```python
from build123d import *

# Parameters (mm, degrees)
SKETCH_1_R          = 100
EXTRUDE_1_DEPTH     = 10
SKETCH_2_W          = 140
SKETCH_2_H          = 100
EXTRUDE_2_DEPTH     = 160.00000000000009
FILLET_1_R          = 70
FILLET_2_R          = 70
SKETCH_3_R          = 50
CUT_EXTRUDE_1_DEPTH = 160.00000000000009
CUT_EXTRUDE_START   = -1
SKETCH_13_R         = 9.999999999999998
CUT_EXTRUDE_5_DEPTH = 25
SKETCH_9_W          = 53.30531277978001
SKETCH_9_H          = 9.28529014360771
EXTRUDE_3_DEPTH     = 100
SKETCH_14_R         = 50
CUT_EXTRUDE_6_DEPTH = 7.7
SKETCH_15_W         = 17.036633895131082
SKETCH_15_H         = 20
CUT_EXTRUDE_7_DEPTH = 110.00000000000001
SKETCH_16_R         = 2.0000000000000036
SKETCH_16_R_2       = 2.000000000000005
SKETCH_16_R_3       = 2.0000000000000013
SKETCH_16_R_4       = 2.0000000000000027
SKETCH_16_R_5       = 2.0000000000000044
CUT_EXTRUDE_8_DEPTH = 10


with BuildPart() as part:
    # 草图1 → 凸台-拉伸1 (new body)
    with BuildSketch(Plane(origin=(0, 0, 0), x_dir=(1, 0, 0), z_dir=(0, 1, 0))):
        with Locations(Location((0, 0, 0), (0, 0, 270))):
            Circle(SKETCH_1_R)
    extrude(amount=EXTRUDE_1_DEPTH)

    # 草图2 → 凸台-拉伸2 (add)
    with BuildSketch(Plane(origin=(0, 0, 0), x_dir=(1, 0, 0), z_dir=(0, 1, 0))):
        Rectangle(SKETCH_2_W, SKETCH_2_H)
    extrude(amount=-EXTRUDE_2_DEPTH)

    # 圆角1
    fillet_1_edges = [part.edges().sort_by_distance(p)[0] for p in [
        (-70.00000000000001, -160.00000000000009, 7.11e-15),
    ]]
    fillet(fillet_1_edges, radius=FILLET_1_R)

    # 圆角2
    fillet_2_edges = [part.edges().sort_by_distance(p)[0] for p in [
        (69.99999999999999, -160.00000000000009, 7.11e-15),
    ]]
    fillet(fillet_2_edges, radius=FILLET_2_R - 0.0001)  # a hair under: the kernel refuses the full size

    # 草图3 → 切除-拉伸1 (cut)
    with BuildSketch(Plane(origin=(0, 0, -49.99999999999999), x_dir=(-1, 0, 0), z_dir=(0, 0, -1))):
        with Locations((0, -90)):
            Circle(SKETCH_3_R)
    extrude(amount=-CUT_EXTRUDE_1_DEPTH, mode=Mode.SUBTRACT)

    # 草图13 → 切除-拉伸5 (cut)
    with BuildSketch(Plane.ZY.offset(70.00000000000001).offset(CUT_EXTRUDE_START)):
        with Locations((6.94e-15, -90.00000000000009)):
            Circle(SKETCH_13_R)
    extrude(amount=-CUT_EXTRUDE_5_DEPTH, mode=Mode.SUBTRACT)

    # 草图9 → 凸台-拉伸3 (add)
    with BuildSketch(Plane(origin=(0, 0, -49.99999999999999), x_dir=(-1, 0, 0), z_dir=(0, 0, -1))):
        with Locations((0.3436291461197136, -140.89264507180383)):
            Rectangle(SKETCH_9_W, SKETCH_9_H)
        Polygon((-23.87404930056264, -43.75), (22.298543315194763, -43.75), (22.298543315194763, -37.81707315136096), (-23.87404930056264, -37.817073151360965), align=None)
    extrude(amount=-EXTRUDE_3_DEPTH)

    # 草图14 → 切除-拉伸6 (cut)
    with BuildSketch(Plane(origin=(0, 0, -49.99999999999999), x_dir=(-1, 0, 0), z_dir=(0, 0, -1))):
        with Locations((0, -90)):
            Circle(SKETCH_14_R)
    extrude(amount=-CUT_EXTRUDE_6_DEPTH, mode=Mode.SUBTRACT)

    # 草图15 → 切除-拉伸7 (cut)
    with BuildSketch(Plane(origin=(0, 10, 0), x_dir=(1, 0, 0), z_dir=(0, 1, 0))):
        with Locations((-60.48168305243448, -7.11e-15)):
            Rectangle(SKETCH_15_W, SKETCH_15_H)
    extrude(amount=-CUT_EXTRUDE_7_DEPTH, mode=Mode.SUBTRACT)

    # 草图16 → 切除-拉伸8 (cut)
    with BuildSketch(Plane(origin=(0, 10, 0), x_dir=(1, 0, 0), z_dir=(0, 1, 0))):
        with Locations(Location((10.537986720028217, 13.656988536588477, 0), (0, 0, 270))):
            Circle(SKETCH_16_R)
        with Locations(Location((17.09629237189259, -2.2976699359932877, 0), (0, 0, 270))):
            Circle(SKETCH_16_R_2)
        with Locations(Location((6.558305651864305, -15.954658472581762, 0), (0, 0, 270))):
            Circle(SKETCH_16_R_3)
        with Locations(Location((-10.537986720028309, -13.656988536588404, 0), (0, 0, 270))):
            Circle(SKETCH_16_R_4)
        with Locations(Location((-17.09629237189257, 2.2976699359934125, 0), (0, 0, 270))):
            Circle(SKETCH_16_R_4)
        with Locations(Location((-6.558305651864193, 15.954658472581803, 0), (0, 0, 270))):
            Circle(SKETCH_16_R_5)
    extrude(amount=-CUT_EXTRUDE_8_DEPTH, mode=Mode.SUBTRACT)


solid = part.part
```
Source: CAD feature listing. Evaluate the final solid. Frame: model axes, mm. A direction names the side the tool comes from. Give positions to 0.01 mm unless a question says otherwise; leave off trailing zeros. Loops run counter-clockwise (first coordinate to the right, second up) from the corner with the lowest first, then second, coordinate; pieces in that order, holes last. Notation, with made-up numbers: (39.5, -8) -> (88.5, -8) arc R31 cw to (88.5, 24) -> close; hole circle Ø5 at (76, 88). An arc over 180 degrees is marked (long way). Use a Markdown table: item, result. Add a question column.
(1) Ray query, line 1 (Z direction, x = -50.7, y = -90); line 2 (Y direction, x = 17, z = 68); line 3 (Y direction, x = -49.7, z = 0). Return the intervals inside material, ascending.
(2) Pull-direction query (Y, two-part tool) for faces 1 (the face through (32, -43, -50)), 2 (the face through (-51, -90, -10)), 3 (the face through (0, -43.75, 3)), 4 (the face through (1, 10, -1)); classes: +Y half, -Y half, draft (parallel to the pull), parting line (faces both ways), or undercut.
(3) Section query B-B (x = 39). Output: boundary loops of the cut face in (y, z), then the cut area to 3 significant figures.
(4) First-contact query: pin 1 Ø2.5 at (x, z) = (-17.1, -2.3) entering from +Y; pin 2 Ø10 at (y, z) = (-118, -33.5) entering from +X; pin 3 Ø3 at (x, y) = (27.5, -130) entering from -Z. Flat tips, straight axial feed; report the tip coordinate or a pass-through.
(5) Access query for faces 5 (the face through (70, -44, 1)), 6 (the face through (-1, -43, 50)), 7 (the face through (0, -136.25, 3)), 8 (the face through (-61, -100, 0)). Directions: +Z, -Z, +X, -X, +Y, -Y. A direction counts if a zero-diameter tool reaches every point of the face in a straight line with its end or side. Return the directions, or none.
(6) Section query A-A (y = -36). Output: boundary loops of the cut face in (x, z), then the cut area to 3 significant figures.
(7) Section query D-D (y = -106.5). Output: boundary loops of the cut face in (x, z).
Checked values:
| question | item | result |
|---|---|---|
| 1 | line 1 | -50 to -10, 10 to 50 |
| 1 | line 2 | 0 to 10 |
| 1 | line 3 | -139.29 to -100, -80 to 10 |
| 2 | face 1 | draft |
| 2 | face 2 | undercut |
| 2 | face 3 | undercut |
| 2 | face 4 | +Y half |
| 3 | outline | (-148.13, -50) -> (-121.29, -50) -> (-121.29, 50) -> (-148.13, 50) -> close; (-58.71, -50) -> (0, -50) -> (0, -92.08) -> (10, -92.08) -> (10, 92.08) -> (0, 92.08) -> (0, 50) -> (-58.71, 50) -> close |
| 3 | area | 10,400 mm^2 |
| 4 | pin 1 | y = 0 |
| 4 | pin 2 | x = 66.11 |
| 4 | pin 3 | z = -50 |
| 5 | face 5 | +Z, -Z, +X, -Y |
| 5 | face 6 | +Z, +X, -X, -Y |
| 5 | face 7 | +Z, -Z |
| 5 | face 8 | +Y |
| 6 | outline | (-70, -50) -> (70, -50) -> (70, 50) -> (-70, 50) -> close; hole (-69, -10) -> (-51.96, -10) -> (-51.96, 10) -> (-69, 10) -> close |
| 6 | area | 13,700 mm^2 |
| 7 | outline | (-68.03, -50) -> (-47.2, -50) -> (-47.2, 50) -> (-68.03, 50) -> close; (47.2, -50) -> (68.03, -50) -> (68.03, 50) -> (47.2, 50) -> close |
